Geometry: final body of the model. Coordinates: model frame, mm. Round coordinates to 2 decimals unless told otherwise and drop trailing zeros. Write each loop counter-clockwise with the first axis right and the second up, starting at its lowest first coordinate (ties: lowest second). Pieces come first, ordered by that corner, then holes. Notation, with made-up numbers: M 73,-24 L 117,-24 A27 cw 117,-4 Z; hole C -10.5,25 d3. An arc over 180 degrees is marked long. Use one line per item in the form item = value. Start each with the question number.
Item 1: Pin query (flat end, axial travel): pin 1 Ø3 at (x, z) = (27.9, 0) entering from +Y; pin 2 Ø2 at (x, z) = (13.44, -14.88) entering from -Y. Return the tip coordinate at first contact, or that it passes through.
Item 2: Section query C-C (z = -10.25). Return loops of the section in (x, y), and give its area (3 significant figures).
Item 3: Ray query, probe 1 along X at (y, z) = (1.3, 0); probe 2 along Z at (x, y) = (13.5, 1.65); probe 3 along X at (y, z) = (0.7, -1). Return the intervals inside material, ascending.
Item 4: Section query B-B (x = 0). Return loops of the section in (y, z).
Item 5: Section query D-D (y = 1.35). Return loops of the section in (x, z).
Item 6: Section query A-A (z = 0). Return loops of the section in (x, y).
from build123d import *

# Parameters (mm, degrees)
SKETCH_1_R      = 1.15
SKETCH_1_R_2    = 0.5
EXTRUDE_1_DEPTH = 2
FILLET_1_R      = 6
FILLET_2_R      = 1.5


with BuildPart() as part:
    # Эскиз1 → Бобышка-Вытянуть1 (new body)
    with BuildSketch(Plane(origin=(0, 0, 0), x_dir=(1, 0, 0), z_dir=(0, 1, 0))):
        with BuildLine():
            Line((25.663932023, -2), (2.236067977, -2))
            ThreePointArc((2.236067977, -2), (-2.74154128, -1.218175444), (0.014385141, 2.999965511))
            Line((0.014385141, 2.999965511), (10.455183999, 14.561088615))
            ThreePointArc((10.455183999, 14.561088615), (13.383244259, 17.879619162), (16.430840693, 14.670516819))
            Line((16.430840693, 14.670516819), (27.775788612, 2.997427486))
            ThreePointArc((27.775788612, 2.997427486), (30.663385612, -1.167775647), (25.663932023, -2))
        make_face()
        with Locations(Location((0, 0, 0), (0, 0, 270))):
            Circle(SKETCH_1_R, mode=Mode.SUBTRACT)
        with Locations(Location((27.9, 0, 0), (0, 0, 270))):
            Circle(SKETCH_1_R, mode=Mode.SUBTRACT)
        with Locations(Location((13.438172043, 14.880122047, 0), (0, 0, 270))):
            Circle(SKETCH_1_R, mode=Mode.SUBTRACT)
        with Locations(Location((24.67605012, 1.362404921, 0), (0, 0, 270))):
            Circle(SKETCH_1_R_2, mode=Mode.SUBTRACT)
        Polygon((13.491730689, 11.955390865), (4.501061475, 2), (23.167266244, 2), align=None, mode=Mode.SUBTRACT)
    extrude(amount=EXTRUDE_1_DEPTH)

    # Скругление1
    fillet_1_edges = [part.edges().sort_by_distance(p)[0] for p in [
        (10.455183999, 1, -14.561088615),
        (16.430840693, 1, -14.670516819),
        (27.775788612, 1, -2.997427486),
        (25.663932023, 1, 2),
        (2.236067977, 1, 2),
        (0.014385141, 1, -2.999965511),
    ]]
    fillet(fillet_1_edges, radius=FILLET_1_R)

    # Скругление2
    fillet_2_edges = [part.edges().sort_by_distance(p)[0] for p in [
        (4.501061475, 1, -2),
        (23.167266244, 1, -2),
        (13.491730689, 1, -11.955390865),
    ]]
    fillet(fillet_2_edges, radius=FILLET_2_R)


solid = part.part
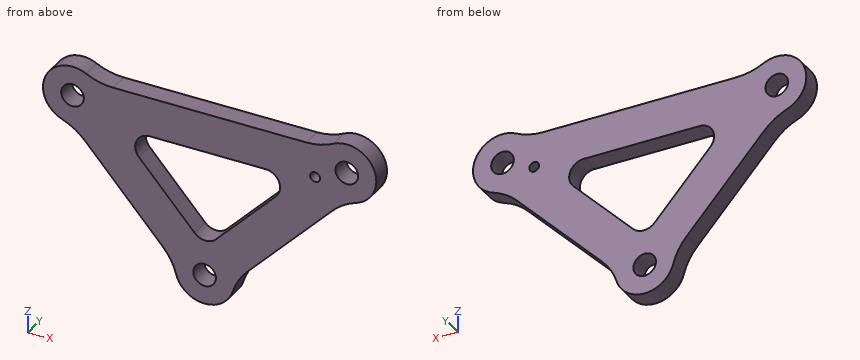
Working result:
q1.pin_1 = 2
q1.pin_2 = through
q2.outline = M 6.56,0 L 11.95,0 L 11.95,2 L 6.56,2 Z; M 15.15,0 L 20.73,0 L 20.73,2 L 15.15,2 Z
q2.area = 21.9 mm²
q3.probe_1 = -3 to -1.15, 1.15 to 26.75, 29.05 to 30.9
q3.probe_2 = -17.88 to -16.03, -13.73 to -11.26, -2 to 2
q3.probe_3 = -2.83 to -0.57, 0.57 to 24.33, 25.02 to 27.33, 28.47 to 30.73
q4.outline = M 0,-3.33 L 2,-3.33 L 2,-1.15 L 0,-1.15 Z; M 0,1.15 L 2,1.15 L 2,3 L 0,3 Z
q5.outline = M -1.06,-2.81 A6 cw 1.28,-4.4 L 9.19,-13.16 A6 cw 10.54,-15.65 A3 ccw 16.31,-15.75 A6 cw 17.75,-13.32 L 26.46,-4.35 A6 cw 28.85,-2.84 A3 ccw long 26.53,2.67 A6 cw 23.78,2 L 4.12,2 A6 cw 1.37,2.67 A3 ccw long Z; hole C 0,0 d2.3; hole M 6.76,-4.51 L 12.42,-10.77 A1.5 ccw 14.61,-10.81 L 20.69,-4.55 A1.5 ccw 19.62,-2 L 7.88,-2 A1.5 ccw Z; hole C 13.44,-14.88 d2.3; hole C 24.68,-1.36 d1; hole C 27.9,0 d2.3
q6.outline = M -3,0 L -1.15,0 L -1.15,2 L -3,2 Z; M 1.15,0 L 26.75,0 L 26.75,2 L 1.15,2 Z; M 29.05,0 L 30.9,0 L 30.9,2 L 29.05,2 Z
